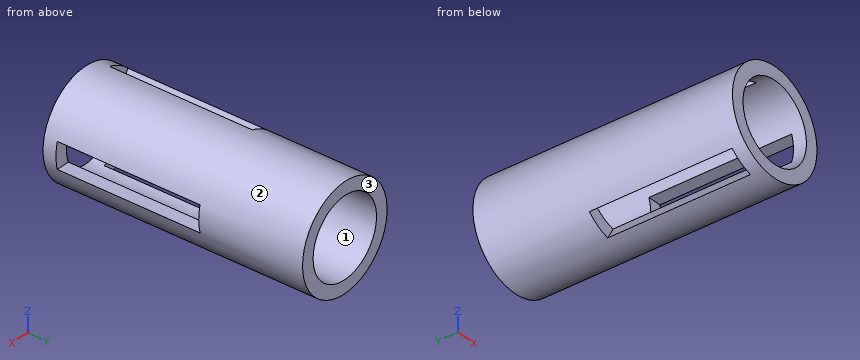
from build123d import *

# Parameters (mm, degrees)
SKETCH1_R           = 20
SKETCH1_R_2         = 15
BOSS_EXTRUDE1_DEPTH = 100
SKETCH2_W           = 10
SKETCH2_H           = 55
CUT_EXTRUDE2_DEPTH  = 5.857864
CIRPATTERN1_COUNT   = 3


with BuildPart() as part:
    # Sketch1 → Boss-Extrude1 (new body)
    with BuildSketch(Plane(origin=(0, 0, 0), x_dir=(1, 0, 0), z_dir=(0, 1, 0))):
        Circle(SKETCH1_R)
        Circle(SKETCH1_R_2, mode=Mode.SUBTRACT)
    extrude(amount=BOSS_EXTRUDE1_DEPTH)

    # Sketch2 → Cut-Extrude2 (cut)
    with BuildSketch(Plane(origin=(20, 0, 0), x_dir=(0, 0, -1), z_dir=(1, 0, 0))):
        with Locations((0, 32.5)):
            Rectangle(SKETCH2_W, SKETCH2_H)
    cut_extrude2 = extrude(amount=-CUT_EXTRUDE2_DEPTH, mode=Mode.SUBTRACT)

    # CirPattern1: Cut-Extrude2 ×3 about axis
    cirpattern1_axis = Axis((0, 0, 0), (0, 1, 0))
    for i in range(1, CIRPATTERN1_COUNT):
        add(cut_extrude2.rotate(cirpattern1_axis, i * 360 / CIRPATTERN1_COUNT), mode=Mode.SUBTRACT)


solid = part.part
Can you work these out from the model? Positions are in its coordinate system, mm. Face numbers are marked on the shaded views. Round coordinates to 2 decimals unless told otherwise and drop trailing zeros. Loops run counter-clockwise (first coordinate to the right, second up) from the corner with the lowest first, then second, coordinate; pieces in that order, holes last. Notation, with made-up numbers: (79.5, 35.25) - (84.5, 35.25) arc R16 cw to (84.5, 45.25) - close; hole circle Ø1 at (-8, 6). An arc over 180 degrees is marked (long way). Write item = value, one per line. Start each with the question number.
(1) If I drill on probe 1 along Z at (x, y) = (0, 65.5); probe 2 along X at (y, z) = (20, 0); probe 3 along Z at (x, y) = (13.5, 27), over which ranges is the centre line in solid material (lowest first)? Write a range as [from, to].
(2) If we section it at A-A (x = 0): Please give me the cut outline in (y, z), and give its area (3 significant figures).
(3) If we section it at C-C (z = 0): Please give me the cut outline in (x, y).
(4) If we mould it in two halves opening along Z, with no side actions, what happens to the marked faces 1, 2 and 3? For each: released by +Z, released by -Z, zero draft, split by the parting line, or undercut.
(5) If we section it at D-D (z = 11.5): Please give me the cut outline in (x, y).
(6) If we section it at B-B (y = 12.5): Please give me the cut outline in (x, z), and give its area (3 significant figures).
(7) For P1, Ø2, axis at x = 4, y = 75.5, coming from the +Z side; P2, Ø5.5, axis at x = 16, y = 24.5, coming from the +Z side; P3, Ø1.5, axis at x = -1, y = 17.5, coming from the +Z side; P4, Ø4, axis at x = -7.5, y = 15, coming from the -Z side, each with a flat end and sliding along its axis, tell me the tip position at first contact or that it passes through.
Ans:
q1.probe_1 = [-20, -15], [15, 20]
q1.probe_2 = [-20, -15]
q1.probe_3 = [-14.76, -6.54], [6.54, 14.76]
q2.outline = (0, -20) - (100, -20) - (100, -15) - (0, -15) - close; (0, 15) - (100, 15) - (100, 20) - (0, 20) - close
q2.area = 1,000 mm²
q3.outline = (-20, 0) - (-15, 0) - (-15, 100) - (-20, 100) - close; (15, 0) - (20, 0) - (20, 5) - (15, 5) - close; (15, 60) - (20, 60) - (20, 100) - (15, 100) - close
q4.face_1 = undercut
q4.face_2 = split by the parting line
q4.face_3 = zero draft
q5.outline = (-16.36, 0) - (-9.63, 0) - (-9.63, 5) - (-12.41, 5) - (-12.41, 60) - (-9.63, 60) - (-9.63, 100) - (-16.36, 100) - close; (9.63, 0) - (16.36, 0) - (16.36, 100) - (9.63, 100) - close
q6.outline = (-14.01, -14.27) - (-11.4, -9.75) arc R15 cw to (-11.4, 9.75) - (-14.01, 14.27) arc R20 ccw to start; (-5.35, -19.27) arc R20 ccw to (19.36, -5) - (14.14, -5) arc R15 cw to (-2.74, -14.75) - close; (-5.35, 19.27) - (-2.74, 14.75) arc R15 cw to (14.14, 5) - (19.36, 5) arc R20 ccw to start
q6.area = 398 mm²
q7.P1 = 19.77
q7.P2 = 14.98
q7.P3 = 20
q7.P4 = through
